from build123d import *

# Parameters (mm, degrees)
F0_W     = 145
F0_H     = 26
F0_W_2   = 2.8837425812
F0_H_2   = 24.8132200628
F1_DEPTH = 25


with BuildPart() as f1:
    # F0 (on Top) → F1 (new body)
    with BuildSketch(Plane.XY):
        with Locations((13.2160319388, 13)):
            Rectangle(F0_W, F0_H)
        with Locations((-49.1691383017, 12.881589666)):
            Rectangle(F0_W_2, F0_H_2, mode=Mode.SUBTRACT)
        with BuildLine():
            Line((-32.417906679, 9.3325769037), (-26.7481755025, 25.2881996974))
            Line((-26.7481755025, 25.2881996974), (-23.6472018417, 25.2881996974))
            Line((-23.6472018417, 25.2881996974), (-32.5862607657, 0.4749796346))
            Line((-32.5862607657, 0.4749796346), (-35.4374186849, 0.4749796346))
            Line((-35.4374186849, 0.4749796346), (-44.3330313929, 25.2881996974))
            Line((-44.3330313929, 25.2881996974), (-41.2755039481, 25.2881996974))
            Line((-41.2755039481, 25.2881996974), (-35.5731881096, 9.2348229179))
            add(Edge.make_bspline(
                [(-35.5731881096, 9.2348229179), (-34.5902174746, 6.4651266535), (-34.0145551138, 3.8529229218)],
                knots=[0, 0, 0, 1, 1, 1], degree=2))
            add(Edge.make_bspline(
                [(-34.0145551138, 3.8529229218), (-33.400877314, 6.6008960782), (-32.417906679, 9.3325769037)],
                knots=[0, 0, 0, 1, 1, 1], degree=2))
        make_face(mode=Mode.SUBTRACT)
        with Locations((-18.7948026021, 12.881589666)):
            Rectangle(F0_W_2, F0_H_2, mode=Mode.SUBTRACT)
        Polygon((-2.3151098289, 13.5414290702), (5.9668250794, 0.4749796346), (2.692066555, 0.4749796346), (-3.9769275875, 11.3854106055), (-10.7653988238, 0.4749796346), (-13.8229262686, 0.4749796346), (-5.5735760223, 13.4436750844), (-13.2635562387, 25.2881996974), (-10.0702593692, 25.2881996974), (-3.9117582636, 15.4584933473), (2.3010506118, 25.2881996974), (5.3694396106, 25.2881996974), align=None, mode=Mode.SUBTRACT)
        with BuildLine():
            add(Edge.make_bspline(
                [(21.1730006487, 23.9875286086), (23.1769573576, 22.3338570154), (23.1769573576, 19.4501144342)],
                knots=[0, 0, 0, 1, 1, 1], degree=2))
            add(Edge.make_bspline(
                [(23.1769573576, 19.4501144342), (23.1769573576, 17.071434113), (21.8437016068, 15.5616781101)],
                knots=[0, 0, 0, 1, 1, 1], degree=2))
            add(Edge.make_bspline(
                [(21.8437016068, 15.5616781101), (20.510445856, 14.0519221071), (18.0665962109, 13.5414290702)],
                knots=[0, 0, 0, 1, 1, 1], degree=2))
            Line((18.0665962109, 13.5414290702), (18.0665962109, 13.4056596454))
            add(Edge.make_bspline(
                [(18.0665962109, 13.4056596454), (21.0535235549, 13.0363668102), (22.4953948455, 11.5076030878)],
                knots=[0, 0, 0, 1, 1, 1], degree=2))
            add(Edge.make_bspline(
                [(22.4953948455, 11.5076030878), (23.9372661361, 9.9788393654), (23.9372661361, 7.5024050584)],
                knots=[0, 0, 0, 1, 1, 1], degree=2))
            add(Edge.make_bspline(
                [(23.9372661361, 7.5024050584), (23.9372661361, 3.9561076845), (21.47712416, 2.0444741844)],
                knots=[0, 0, 0, 1, 1, 1], degree=2))
            add(Edge.make_bspline(
                [(21.47712416, 2.0444741844), (19.016982184, 0.1328406843), (14.4877141752, 0.1328406843)],
                knots=[0, 0, 0, 1, 1, 1], degree=2))
            add(Edge.make_bspline(
                [(14.4877141752, 0.1328406843), (12.5163421282, 0.1328406843), (10.878962866, 0.4315334187)],
                knots=[0, 0, 0, 1, 1, 1], degree=2))
            add(Edge.make_bspline(
                [(10.878962866, 0.4315334187), (9.2415836038, 0.7302261531), (7.6992429389, 1.4742426006)],
                knots=[0, 0, 0, 1, 1, 1], degree=2))
            Line((7.6992429389, 1.4742426006), (7.6992429389, 4.1570464331))
            add(Edge.make_bspline(
                [(7.6992429389, 4.1570464331), (9.3121837046, 3.3587222158), (11.1369247729, 2.9432677761)],
                knots=[0, 0, 0, 1, 1, 1], degree=2))
            add(Edge.make_bspline(
                [(11.1369247729, 2.9432677761), (12.9616658413, 2.5278133364), (14.590898938, 2.5278133364)],
                knots=[0, 0, 0, 1, 1, 1], degree=2))
            add(Edge.make_bspline(
                [(14.590898938, 2.5278133364), (21.020938893, 2.5278133364), (21.020938893, 7.5675743822)],
                knots=[0, 0, 0, 1, 1, 1], degree=2))
            add(Edge.make_bspline(
                [(21.020938893, 7.5675743822), (21.020938893, 12.0859808371), (13.9283441453, 12.0859808371)],
                knots=[0, 0, 0, 1, 1, 1], degree=2))
            Line((13.9283441453, 12.0859808371), (11.4844945002, 12.0859808371))
            Line((11.4844945002, 12.0859808371), (11.4844945002, 14.5081073742))
            Line((11.4844945002, 14.5081073742), (13.9609288072, 14.5081073742))
            add(Edge.make_bspline(
                [(13.9609288072, 14.5081073742), (16.8609637194, 14.5081073742), (18.5580815284, 15.7897707436)],
                knots=[0, 0, 0, 1, 1, 1], degree=2))
            add(Edge.make_bspline(
                [(18.5580815284, 15.7897707436), (20.2551993375, 17.071434113), (20.2551993375, 19.3469296714)],
                knots=[0, 0, 0, 1, 1, 1], degree=2))
            add(Edge.make_bspline(
                [(20.2551993375, 19.3469296714), (20.2551993375, 21.1608091858), (19.0088360185, 22.1980875907)],
                knots=[0, 0, 0, 1, 1, 1], degree=2))
            add(Edge.make_bspline(
                [(19.0088360185, 22.1980875907), (17.7624726995, 23.2353659956), (15.6227465659, 23.2353659956)],
                knots=[0, 0, 0, 1, 1, 1], degree=2))
            add(Edge.make_bspline(
                [(15.6227465659, 23.2353659956), (13.9935134692, 23.2353659956), (12.5516421786, 22.792757671)],
                knots=[0, 0, 0, 1, 1, 1], degree=2))
            add(Edge.make_bspline(
                [(12.5516421786, 22.792757671), (11.109770888, 22.3501493464), (9.2578759347, 21.1608091858)],
                knots=[0, 0, 0, 1, 1, 1], degree=2))
            Line((9.2578759347, 21.1608091858), (7.8350123636, 23.0615811319))
            add(Edge.make_bspline(
                [(7.8350123636, 23.0615811319), (9.3610606975, 24.2672136235), (11.3541558525, 24.9542069126)],
                knots=[0, 0, 0, 1, 1, 1], degree=2))
            add(Edge.make_bspline(
                [(11.3541558525, 24.9542069126), (13.3472510075, 25.6412002017), (15.557577242, 25.6412002017)],
                knots=[0, 0, 0, 1, 1, 1], degree=2))
            add(Edge.make_bspline(
                [(15.557577242, 25.6412002017), (19.1690439397, 25.6412002017), (21.1730006487, 23.9875286086)],
                knots=[0, 0, 0, 1, 1, 1], degree=2))
        make_face(mode=Mode.SUBTRACT)
        Polygon((33.9353265729, 0.4749796346), (30.8126298042, 0.4749796346), (41.0930906444, 22.6922882967), (27.5704559417, 22.6922882967), (27.5704559417, 25.2881996974), (44.0800179883, 25.2881996974), (44.0800179883, 23.02899647), align=None, mode=Mode.SUBTRACT)
        with BuildLine():
            Line((57.9773763033, 25.2881996974), (57.9773763033, 0.4749796346))
            Line((57.9773763033, 0.4749796346), (55.2294031468, 0.4749796346))
            Line((55.2294031468, 0.4749796346), (55.2294031468, 18.1575895108))
            add(Edge.make_bspline(
                [(55.2294031468, 18.1575895108), (55.2294031468, 20.3679157454), (55.3651725715, 22.3338570154)],
                knots=[0, 0, 0, 1, 1, 1], degree=2))
            add(Edge.make_bspline(
                [(55.3651725715, 22.3338570154), (55.0121720672, 21.9754257341), (54.5695637426, 21.5871251794)],
                knots=[0, 0, 0, 1, 1, 1], degree=2))
            add(Edge.make_bspline(
                [(54.5695637426, 21.5871251794), (54.126955418, 21.1988246247), (50.5317810513, 18.2770666046)],
                knots=[0, 0, 0, 1, 1, 1], degree=2))
            Line((50.5317810513, 18.2770666046), (49.0383173793, 20.2104232127))
            Line((49.0383173793, 20.2104232127), (55.6041267591, 25.2881996974))
            Line((55.6041267591, 25.2881996974), (57.9773763033, 25.2881996974))
        make_face(mode=Mode.SUBTRACT)
        with BuildLine():
            Line((83.7246900082, 3.0871833663), (83.7246900082, 0.4749796346))
            Line((83.7246900082, 0.4749796346), (67.4160667102, 0.4749796346))
            Line((67.4160667102, 0.4749796346), (67.4160667102, 2.9025369487))
            Line((67.4160667102, 2.9025369487), (73.949291428, 9.4683463284))
            add(Edge.make_bspline(
                [(73.949291428, 9.4683463284), (76.9362187719, 12.4932891113), (77.886604745, 13.7830986462)],
                knots=[0, 0, 0, 1, 1, 1], degree=2))
            add(Edge.make_bspline(
                [(77.886604745, 13.7830986462), (78.8369907181, 15.0729081811), (79.3121837046, 16.2948330036)],
                knots=[0, 0, 0, 1, 1, 1], degree=2))
            add(Edge.make_bspline(
                [(79.3121837046, 16.2948330036), (79.7873766912, 17.5167578261), (79.7873766912, 18.9233290663)],
                knots=[0, 0, 0, 1, 1, 1], degree=2))
            add(Edge.make_bspline(
                [(79.7873766912, 18.9233290663), (79.7873766912, 20.9109934443), (78.5817441996, 22.0731797199)],
                knots=[0, 0, 0, 1, 1, 1], degree=2))
            add(Edge.make_bspline(
                [(78.5817441996, 22.0731797199), (77.376111708, 23.2353659956), (75.2363855744, 23.2353659956)],
                knots=[0, 0, 0, 1, 1, 1], degree=2))
            add(Edge.make_bspline(
                [(75.2363855744, 23.2353659956), (73.6940449095, 23.2353659956), (72.3091967773, 22.7248729586)],
                knots=[0, 0, 0, 1, 1, 1], degree=2))
            add(Edge.make_bspline(
                [(72.3091967773, 22.7248729586), (70.9243486451, 22.2143799216), (69.2299462245, 20.8729780054)],
                knots=[0, 0, 0, 1, 1, 1], degree=2))
            Line((69.2299462245, 20.8729780054), (67.7364825525, 22.7900422825))
            add(Edge.make_bspline(
                [(67.7364825525, 22.7900422825), (71.1633028326, 25.6412002017), (75.2038009124, 25.6412002017)],
                knots=[0, 0, 0, 1, 1, 1], degree=2))
            add(Edge.make_bspline(
                [(75.2038009124, 25.6412002017), (78.7012212934, 25.6412002017), (80.6861702829, 23.8517591838)],
                knots=[0, 0, 0, 1, 1, 1], degree=2))
            add(Edge.make_bspline(
                [(80.6861702829, 23.8517591838), (82.6711192723, 22.0623181659), (82.6711192723, 19.0428061601)],
                knots=[0, 0, 0, 1, 1, 1], degree=2))
            add(Edge.make_bspline(
                [(82.6711192723, 19.0428061601), (82.6711192723, 16.6804181698), (81.346009687, 14.3723379495)],
                knots=[0, 0, 0, 1, 1, 1], degree=2))
            add(Edge.make_bspline(
                [(81.346009687, 14.3723379495), (80.0209001017, 12.0642577292), (76.393141073, 8.5342526863)],
                knots=[0, 0, 0, 1, 1, 1], degree=2))
            Line((76.393141073, 8.5342526863), (70.962364084, 3.222952791))
            Line((70.962364084, 3.222952791), (70.962364084, 3.0871833663))
            Line((70.962364084, 3.0871833663), (83.7246900082, 3.0871833663))
        make_face(mode=Mode.SUBTRACT)
    extrude(amount=F1_DEPTH)


solid = f1.part
Geometry: final body of the model. Coordinates: model frame, mm. A direction names the side the tool comes from. Give positions to 0.01 mm unless a question says otherwise; leave off trailing zeros. Loops run counter-clockwise (first coordinate to the right, second up) from the corner with the lowest first, then second, coordinate; pieces in that order, holes last. Notation, with made-up numbers: M 44,50 L 73,50 A30 ccw 73,76 Z; hole C 81,54.25 d5. An arc over 180 degrees is marked long. Put each result on its own line as item: value. Start each with the question number.
1) Pull-direction query (X, two-part tool) for faces 3 (the flat face through (-59.284, 13, 12)), 4 (the flat face through (85.716, 13, 12)), 5 (the flat face through (39.08, 11.91, 12.32)); classes: pulls with the +X half, pulls with the -X half, needs draft (parallel to the pull), parting line crosses it, or undercut.
2) Ray query, line 1 along Y through (x, z) = (21.5, 14.5); line 2 along Y through (x, z) = (-11.5, 15.25); line 3 along Y through (x, z) = (16, 11.25). Return the intervals inside material, ascending.
3) Cut plane C-C (x = -30). Output: boundary loops of the cut face in (y, z).
4) Cut plane B-B (z = 19). Give the number of separate pieces and of enclosed holes in the cut face, then the cut area to 3 significant figures.
5) Cut plane A-A (x = -49). Output: boundary loops of the cut face in (y, z), then the cut area to 3 significant figures.
6) Access query for faces 1 (the flat face through (12, 0, 12)), 2 (the flat face through (-9.365, 19.283, 12.325)). Directions: +Z, -Z, +X, -X, +Y, -Y. A direction counts if a zero-diameter tool reaches every point of the face in a straight line with its end or side. Return the directions, or none.
Verdict:
1. face 3: pulls with the -X half
1. face 4: pulls with the +X half
1. face 5: undercut
2. line 1: 0 to 2.06, 12.32 to 15.21, 23.7 to 26
2. line 2: 0 to 0.47, 4.13 to 22.57, 25.29 to 26
2. line 3: 0 to 0.19, 2.6 to 11.97, 14.69 to 23.23, 25.63 to 26
3. outline: M 0,0 L 7.65,0 L 7.65,25 L 0,25 Z; M 16.14,0 L 26,0 L 26,25 L 16.14,25 Z
4. separate pieces: 1
4. enclosed holes: 8
4. area: 2,870 mm2
5. outline: M 0,0 L 0.47,0 L 0.47,25 L 0,25 Z; M 25.29,0 L 26,0 L 26,25 L 25.29,25 Z
5. area: 29.7 mm2
6. face 1: +Z, -Z, +X, -X, -Y
6. face 2: +Z, -Z
